Part model, mm, in its own coordinate system. A direction names the side the tool comes from. Coordinates: 2 decimals unless noted, no trailing zeros. Write each loop counter-clockwise with the first axis right and the second up, starting at its lowest first coordinate (ties: lowest second). Pieces come first, ordered by that corner, then holes. Notation, with made-up numbers: M 5.5,77 L 62.5,77 A19 cw 62.5,99 Z; hole C 43.25,34 d3. An arc over 180 degrees is marked long. Use a Markdown table: item, result. Add a question column.
Q1. Wall check: L1, parallel to X at y = 1.65, z = 0; L2, parallel to X at y = 23, z = 12.5; L3, parallel to Y at x = 13.5, z = 3. Give the ranges that are in metal, low to high. Write a range as from..to.
Q2. Pin check, flat tips, straight feed: pin 1 Ø5 at (x, z) = (5.5, 22.5) entering from +Y; pin 2 Ø4 at (x, y) = (-11.5, 1.5) entering from +Z; pin 3 Ø1.5 at (y, z) = (15, 19) entering from -X; pin 4 Ø10 at (y, z) = (6, 16.5) entering from -X. Stop position of each tip, or through.
Q3. Slice it at B-B on z = 23. Write the cut outline in (x, y).
Q4. Slice it at D-D on y = 21. Write the cut outline in (x, z), then the cut area to 3 significant figures.
Q5. Slice it at A-A on z = 0. Write the cut outline in (x, y).
Q6. Slice it at C-C on z = 10.5. Write the cut outline in (x, y), then the cut area to 3 significant figures.
Q7. Tool access for faces 1 (the flat face through (-9, 5.08, 1)), 2 (the flat face through (-11, 3, 7.62)), 3 (the flat face through (9, 5.08, 1)): list every direction of +Z, -Z, +X, -X, +Y, -Y with a clear straight run to the whole face (end or side of a thin tool).
from build123d import *

# Parameters (mm, degrees)
SKETCH1_R           = 2.0828
BOSS_EXTRUDE1_DEPTH = 5.08
SKETCH2_R           = 1.7526
BOSS_EXTRUDE2_DEPTH = 2.54
FILLET1_R           = 6.35


with BuildPart() as part:
    # Sketch1 → Boss-Extrude1 (new body)
    with BuildSketch(Plane(origin=(0, 0, 0), x_dir=(1, 0, 0), z_dir=(0, 1, 0))):
        with BuildLine():
            Line((-12.7, -7.62), (12.7, -7.62))
            ThreePointArc((12.7, -7.62), (17.190128061, -5.760128061), (19.05, -1.27))
            Line((19.05, -1.27), (19.05, 1.27))
            ThreePointArc((19.05, 1.27), (17.190128061, 5.760128061), (12.7, 7.62))
            Line((12.7, 7.62), (-12.7, 7.62))
            ThreePointArc((-12.7, 7.62), (-17.190128061, 5.760128061), (-19.05, 1.27))
            Line((-19.05, 1.27), (-19.05, -1.27))
            ThreePointArc((-19.05, -1.27), (-17.190128061, -5.760128061), (-12.7, -7.62))
        make_face()
        with Locations(Location((-12.7, 0, 0), (0, 0, 270))):
            Circle(SKETCH1_R, mode=Mode.SUBTRACT)
        with Locations(Location((12.7, 0, 0), (0, 0, 270))):
            Circle(SKETCH1_R, mode=Mode.SUBTRACT)
    extrude(amount=BOSS_EXTRUDE1_DEPTH)

    # Sketch2 → Boss-Extrude2 (add, symmetric)
    with BuildSketch(Plane(origin=(0, 0, 0), x_dir=(0, 0, -1), z_dir=(1, 0, 0))):
        with BuildLine():
            Line((7.62, 5.08), (-17.785245966, 34.910144211))
            ThreePointArc((-17.785245966, 34.910144211), (-25.347393839, 36.891939152), (-29.8196, 30.48))
            Line((-29.8196, 30.48), (-29.8196, 0))
            Line((-29.8196, 0), (7.62, 0))
            Line((7.62, 0), (7.62, 5.08))
        make_face()
        with Locations((-22.987, 30.48)):
            Circle(SKETCH2_R, mode=Mode.SUBTRACT)
    extrude(amount=BOSS_EXTRUDE2_DEPTH, both=True)

    # Fillet1
    fillet1_edges = [part.edges().sort_by_distance(p)[0] for p in [
        (-2.54, 2.54, 7.62),
        (2.54, 2.54, 7.62),
    ]]
    fillet(fillet1_edges, radius=FILLET1_R)


solid = part.part
Recorded:
| question | item | result |
|---|---|---|
| 1 | L1 | -19.05..-14.78, -10.62..10.62, 14.78..19.05 |
| 1 | L2 | -2.54..2.54 |
| 1 | L3 | 0..5.08 |
| 2 | pin 1 | through |
| 2 | pin 2 | z = 7.62 |
| 2 | pin 3 | x = -2.54 |
| 2 | pin 4 | x = -3 |
| 3 | outline | M -2.54,0 L 2.54,0 L 2.54,28.73 L -2.54,28.73 Z; M -2.54,32.23 L 2.54,32.23 L 2.54,37.31 L -2.54,37.31 Z |
| 4 | outline | M -2.54,5.94 L 2.54,5.94 L 2.54,29.82 L -2.54,29.82 Z |
| 4 | area | 121 mm² |
| 5 | outline | M -19.05,0 L -14.78,0 L -14.78,5.08 L -19.05,5.08 Z; M -10.62,0 L 10.62,0 L 10.62,5.08 L 2.54,5.08 L 2.54,14.03 L -2.54,14.03 L -2.54,5.08 L -10.62,5.08 Z; M 14.78,0 L 19.05,0 L 19.05,5.08 L 14.78,5.08 Z |
| 6 | outline | M -3.57,0 L 3.57,0 L 3.57,5.08 L 2.54,5.08 L 2.54,26.36 L -2.54,26.36 L -2.54,5.08 L -3.57,5.08 Z |
| 6 | area | 144 mm² |
| 7 | face 1 | +Z, -Z, -X, +Y |
| 7 | face 2 | +Z, -X, +Y, -Y |
| 7 | face 3 | +Z, -Z, +X, +Y |
